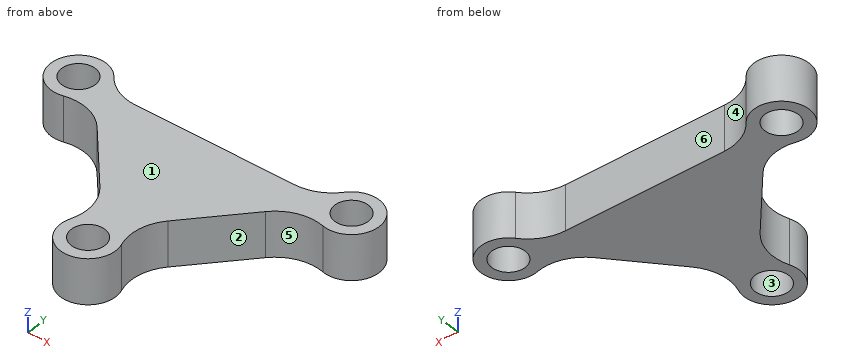
```python
from build123d import *

# Parameters (mm, degrees)
ESQUISSE2_R        = 3
ESQUISSE2_R_2      = 1.825
BOSS_EXTRU_1_DEPTH = 4.89
CONG_1_R           = 5


with BuildPart() as part:
    # Esquisse2 → Boss.-Extru.1 (new body)
    # profile 1 of 4: a face of its own
    with BuildSketch(Plane.XY):
        with Locations((-15, 10)):
            Circle(ESQUISSE2_R)
        with Locations((-15, 10)):
            Circle(ESQUISSE2_R_2, mode=Mode.SUBTRACT)
    # profile 2 of 4: a face of its own
    with BuildSketch(Plane.XY):
        with Locations((15, 10)):
            Circle(ESQUISSE2_R)
        with Locations((15, 10)):
            Circle(ESQUISSE2_R_2, mode=Mode.SUBTRACT)
    # profile 3 of 4: a face of its own
    with BuildSketch(Plane.XY):
        with Locations((0, -6.825)):
            Circle(ESQUISSE2_R)
        with Locations((0, -6.825)):
            Circle(ESQUISSE2_R_2, mode=Mode.SUBTRACT)
    # profile 4 of 4: a face of its own
    with BuildSketch(Plane.XY):
        Polygon((-13.175, 10), (13.175, 10), (0, -5), align=None)
    extrude(amount=BOSS_EXTRU_1_DEPTH)

    # Congé1
    cong_1_edges = [part.edges().sort_by_distance(p)[0] for p in [
        (-12.208908932, 8.900086071, 2.445),
        (-12, 10, 2.445),
        (12, 10, 2.445),
        (12.208908932, 8.900086071, 2.445),
        (0.908352526, -3.965822551, 2.445),
        (-0.908352526, -3.965822551, 2.445),
    ]]
    fillet(cong_1_edges, radius=CONG_1_R)


solid = part.part
```
For this review, take the finished solid that the model builds, in its own axes (mm). Face numbers are marked on the shaded views. A direction names the side the tool comes from. Coordinates: 2 decimals unless noted, no trailing zeros. Write each loop counter-clockwise with the first axis right and the second up, starting at its lowest first coordinate (ties: lowest second). Pieces come first, ordered by that corner, then holes.
(1) For pin 1 Ø1.5 at (x, z) = (3.5, 2.5) entering from +Y; pin 2 Ø3.5 at (x, y) = (-15, 10) entering from -Z, all flat-tipped, find the tip position at first contact; note any pin that passes through.
(2) Add section C-C on x = 0. Give the boundary of the cut face in (y, z) (3 decimals), then the cut area to 3 significant figures.
(3) Wall thickness on probe 1 along Y at (x, z) = (0, 2.95) (3 decimals); probe 2 along Y at (x, z) = (15, 1.1) (3 decimals); probe 3 along Y at (x, z) = (6, 0.75): over which ranges is each line inside the solid? List them lowest first.
(4) Add section B-B on z = 3.1. Give the boundary of the cut face in (x, y) (3 decimals), then the cut area to 3 significant figures.
(5) Tool access review of the marked faces 5 and 6: name each direction out of +Z, -Z, +X, -X, +Y, -Y from which nothing blocks a thin tool from reaching the whole face with its end or side.
(6) The part is to be moulded in two halves that separate along Y. For the marked faces 1, 2, 3 and 4, say which applies: +Y half, -Y half, draft (parallel to the pull), parting line (faces both ways), or undercut.
(7) Add section D-D on y = -1.5. Give the boundary of the cut face in (x, z), then the cut area to 3 significant figures.
(8) Add section A-A on x = -15. Give the boundary of the cut face in (y, z) (3 decimals), then the cut area to 3 significant figures.
Answer sheet:
1. pin 1: stops at y = 10
1. pin 2: passes through
2. outline: (-9.825, 0) - (-8.65, 0) - (-8.65, 4.89) - (-9.825, 4.89) - close; (-5, 0) - (10, 0) - (10, 4.89) - (-5, 4.89) - close
2. area: 79.1 mm2
3. probe 1: y = -9.825 to -8.65, -5 to 10
3. probe 2: y = 7 to 8.175, 11.825 to 13
3. probe 3: y = 1.83 to 10
4. outline: (-14.258, 7.093) arc R5 cw to (-9.265, 5.548) - (-3.742, -0.739) arc R5 cw to (-2.812, -5.78) arc R3 ccw (long way) to (2.812, -5.78) arc R5 cw to (3.742, -0.739) - (9.265, 5.548) arc R5 cw to (14.258, 7.093) arc R3 ccw (long way) to (12.658, 11.875) arc R5 cw to (8.755, 10) - (-8.755, 10) arc R5 cw to (-12.658, 11.875) arc R3 ccw (long way) to start; hole circle Ø3.65 at (-15, 10); hole circle Ø3.65 at (0, -6.825); hole circle Ø3.65 at (15, 10)
4. area: 262 mm2
5. face 5: +Z, -Z, -Y
5. face 6: +Z, -Z, +Y
6. face 1: draft
6. face 2: -Y half
6. face 3: undercut
6. face 4: +Y half
7. outline: (-3.19, 0) - (3.19, 0) - (3.19, 4.89) - (-3.19, 4.89) - close
7. area: 31.2 mm2
8. outline: (7, 0) - (8.175, 0) - (8.175, 4.89) - (7, 4.89) - close; (11.825, 0) - (13, 0) - (13, 4.89) - (11.825, 4.89) - close
8. area: 11.5 mm2
